from build123d import *

# Parameters (mm, degrees)
SKETCH1_W                            = 254
SKETCH1_H                            = 177.8
BOSS_EXTRUDE1_DEPTH                  = 127
SKETCH2_W                            = 241.3
SKETCH2_H                            = 165.1
CUT_EXTRUDE1_DEPTH                   = 101.6
F_3_16_0_1875_DIAMETER_HOLE3_D       = 4.7625
F_3_16_0_1875_DIAMETER_HOLE3_DEPTH   = 12.7
F_3_16_0_1875_DIAMETER_HOLE3_TIP     = 1.430799349
F_3_16_0_1875_DIAMETER_HOLE4_D       = 4.7625
F_3_16_0_1875_DIAMETER_HOLE4_DEPTH   = 12.7
F_3_16_0_1875_DIAMETER_HOLE4_TIP     = 1.430799349
F_3_16_0_1875_DIAMETER_HOLE5_D       = 4.7625
F_3_16_0_1875_DIAMETER_HOLE5_DEPTH   = 12.7
F_3_16_0_1875_DIAMETER_HOLE5_TIP     = 1.430799349
F_3_16_0_1875_DIAMETER_HOLE6_D       = 4.7625
F_3_16_0_1875_DIAMETER_HOLE6_DEPTH   = 12.7
F_3_16_0_1875_DIAMETER_HOLE6_TIP     = 1.430799349
F_11_64_0_17188_DIAMETER_HOLE1_D     = 4.365752
F_11_64_0_17188_DIAMETER_HOLE1_DEPTH = 6.35


with BuildPart() as part:
    # Sketch1 → Boss-Extrude1 (new body)
    with BuildSketch(Plane(origin=(0, 0, 0), x_dir=(1, 0, 0), z_dir=(0, 1, 0))):
        Rectangle(SKETCH1_W, SKETCH1_H)
    extrude(amount=BOSS_EXTRUDE1_DEPTH)

    # Sketch2 → Cut-Extrude1 (cut)
    with BuildSketch(Plane(origin=(0, 127, 0), x_dir=(1, 0, 0), z_dir=(0, 1, 0))):
        Rectangle(SKETCH2_W, SKETCH2_H)
    extrude(amount=-CUT_EXTRUDE1_DEPTH, mode=Mode.SUBTRACT)

    # 3/16 (0.1875) Diameter Hole3
    with Locations(Plane(origin=(-123.698, 127, -85.598), x_dir=(0, 0, 1), z_dir=(0, 1, 0))):
        with Locations((0, 0)):
            Hole(F_3_16_0_1875_DIAMETER_HOLE3_D / 2, depth=F_3_16_0_1875_DIAMETER_HOLE3_DEPTH)
            with Locations((0, 0, -(F_3_16_0_1875_DIAMETER_HOLE3_DEPTH + F_3_16_0_1875_DIAMETER_HOLE3_TIP / 2))):  # 118° drill point
                Cone(0, F_3_16_0_1875_DIAMETER_HOLE3_D / 2, F_3_16_0_1875_DIAMETER_HOLE3_TIP, mode=Mode.SUBTRACT)

    # 3/16 (0.1875) Diameter Hole4
    with Locations(Plane(origin=(123.698, 127, -85.598), x_dir=(0, 0, 1), z_dir=(0, 1, 0))):
        with Locations((0, 0)):
            Hole(F_3_16_0_1875_DIAMETER_HOLE4_D / 2, depth=F_3_16_0_1875_DIAMETER_HOLE4_DEPTH)
            with Locations((0, 0, -(F_3_16_0_1875_DIAMETER_HOLE4_DEPTH + F_3_16_0_1875_DIAMETER_HOLE4_TIP / 2))):  # 118° drill point
                Cone(0, F_3_16_0_1875_DIAMETER_HOLE4_D / 2, F_3_16_0_1875_DIAMETER_HOLE4_TIP, mode=Mode.SUBTRACT)

    # 3/16 (0.1875) Diameter Hole5
    with Locations(Plane(origin=(-123.698, 127, 85.598), x_dir=(0, 0, 1), z_dir=(0, 1, 0))):
        with Locations((0, 0)):
            Hole(F_3_16_0_1875_DIAMETER_HOLE5_D / 2, depth=F_3_16_0_1875_DIAMETER_HOLE5_DEPTH)
            with Locations((0, 0, -(F_3_16_0_1875_DIAMETER_HOLE5_DEPTH + F_3_16_0_1875_DIAMETER_HOLE5_TIP / 2))):  # 118° drill point
                Cone(0, F_3_16_0_1875_DIAMETER_HOLE5_D / 2, F_3_16_0_1875_DIAMETER_HOLE5_TIP, mode=Mode.SUBTRACT)

    # 3/16 (0.1875) Diameter Hole6
    with Locations(Plane(origin=(123.698, 127, 85.598), x_dir=(0, 0, 1), z_dir=(0, 1, 0))):
        with Locations((0, 0)):
            Hole(F_3_16_0_1875_DIAMETER_HOLE6_D / 2, depth=F_3_16_0_1875_DIAMETER_HOLE6_DEPTH)
            with Locations((0, 0, -(F_3_16_0_1875_DIAMETER_HOLE6_DEPTH + F_3_16_0_1875_DIAMETER_HOLE6_TIP / 2))):  # 118° drill point
                Cone(0, F_3_16_0_1875_DIAMETER_HOLE6_D / 2, F_3_16_0_1875_DIAMETER_HOLE6_TIP, mode=Mode.SUBTRACT)

    # 11/64 (0.17188) Diameter Hole1
    with Locations(Plane.XY.offset(-82.55)):
        with Locations((90.000861875, 33.401943058), (90.000861875, 61.115793816), (77.507570052, 52.735678174), (77.507570052, 38.856201142), (103.356898088, 52.735678174), (103.356898088, 38.856201142), (90.000861875, 46.977884259)):
            Hole(F_11_64_0_17188_DIAMETER_HOLE1_D / 2, depth=F_11_64_0_17188_DIAMETER_HOLE1_DEPTH)


solid = part.part
Source: CAD feature listing. Evaluate the final solid. Frame: model axes, mm. A direction names the side the tool comes from. Round coordinates to 2 decimals unless told otherwise and drop trailing zeros. Loops run counter-clockwise (first coordinate to the right, second up) from the corner with the lowest first, then second, coordinate; pieces in that order, holes last. Notation, with made-up numbers: M 50,77 L 95,77 A21 ccw 95,96 Z; hole C 6,49 d9. An arc over 180 degrees is marked long. Answer as CSV lines item,"result".
Q1. Cut plane C-C (x = -73.5). Return the cut outline in (y, z).
Verdict:
outline,"M 0,-88.9 L 127,-88.9 L 127,-82.55 L 25.4,-82.55 L 25.4,82.55 L 127,82.55 L 127,88.9 L 0,88.9 Z"
Q2. Line query: line 1 along Z through (x, y) = (7, 83); line 2 along X through (y, z) = (105.5, 55); line 3 along Y through (x, z) = (37, 0.5). Output: solid intervals per line, ascending.
Verdict:
line 1,"z = -88.9 to -82.55, 82.55 to 88.9"
line 2,"x = -127 to -120.65, 120.65 to 127"
line 3,"y = 0 to 25.4"
Q3. Reachability of faces 1 (the face through (-2, 25.4, -1)), 2 (the face through (-2, 63, -88.9)) from +Z, -Z, +X, -X, +Y, -Y: full face, straight path, thin tool, end or side. Return the list, or none.
Verdict:
face 1,"+Y"
face 2,"-Z, +X, -X, +Y, -Y"
Q4. Cut plane A-A (y = 85). Return the cut outline in (x, z).
Verdict:
outline,"M -127,-88.9 L 127,-88.9 L 127,88.9 L -127,88.9 Z; hole M -120.65,-82.55 L 120.65,-82.55 L 120.65,82.55 L -120.65,82.55 Z"
Q5. Contact query for flat-ended pins moving along their axis: pin 1 (2.5 mm diameter, centred on x = 90, y = 61.12, fed in from -Z); pin 2 (4 mm diameter, centred on x = -63.5, z = -0.5, fed in from +Y). Output: stop coordinate, or through.
Verdict:
pin 1,"stops at z = 82.55"
pin 2,"stops at y = 25.4"
Q6. Pull-direction query (X, two-part tool) for faces 3 (the face through (-2, 77, -82.55)), 4 (the face through (-1, 127, -86)), 5 (the face through (127, 63, 1)); classes: +X half, -X half, draft (parallel to the pull), parting line (faces both ways), or undercut.
Verdict:
face 3,"undercut"
face 4,"draft"
face 5,"+X half"
Q7. Cut plane B-B (z = -41.5). Return the cut outline in (x, y).
Verdict:
outline,"M -127,0 L 127,0 L 127,127 L 120.65,127 L 120.65,25.4 L -120.65,25.4 L -120.65,127 L -127,127 Z"
